Could you check a few things on this model? Use its own coordinates, in mm. Coordinates: 2 decimals unless noted, no trailing zeros. Write each loop counter-clockwise with the first axis right and the second up, starting at its lowest first coordinate (ties: lowest second). Pieces come first, ordered by that corner, then holes.
Autodesk Inventor part; units mm, degrees
ref_plane "YZ Plane" through (0, 0, 0) normal (1, 0, 0) x (0, 1, 0)
ref_plane "XZ Plane" through (0, 0, 0) normal (0, 1, 0) x (-1, 0, 0)
ref_plane "XY Plane" through (0, 0, 0) normal (0, 0, 1) x (1, 0, 0)
sketch "Sketch1" plane through (0, 0, 0) normal (0, 1, 0) x (-1, 0, 0)
  line L0 (2.286, 0) -> (10.414, 0)
  line L1 (12.7, -2.286) -> (12.7, -10.414)
  line L2 (10.414, -12.7) -> (2.286, -12.7)
  line L3 (0, -10.414) -> (0, -2.286)
  line L4 (8.1534, -4.0386) -> (4.5466, -4.0386)
  line L5 (4.0386, -4.5466) -> (4.0386, -8.1534)
  line L6 (4.5466, -8.6614) -> (8.1534, -8.6614)
  line L7 (8.6614, -8.1534) -> (8.6614, -4.5466)
  line L8 (10.414, 0) -> (12.7, -2.286)
  line L9 (12.7, -10.414) -> (10.414, -12.7)
  line L10 (2.286, -12.7) -> (0, -10.414)
  line L11 (2.286, 0) -> (0, -2.286)
  arc A0 (8.6614, -4.5466) -> (8.1534, -4.0386) centre (8.1534, -4.5466) ccw
  arc A1 (8.1534, -8.6614) -> (8.6614, -8.1534) centre (8.1534, -8.1534) ccw
  arc A2 (4.0386, -8.1534) -> (4.5466, -8.6614) centre (4.5466, -8.1534) ccw
  arc A3 (4.5466, -4.0386) -> (4.0386, -4.5466) centre (4.5466, -4.5466) ccw
  line L12 (8.1534, -4.5466) -> (4.5466, -8.1534) construction
  line L13 (12.7, -10.414) -> (0, -2.286) construction
  point P0 (0, 0)
  point P1 (12.7, -12.7)
  point P2 (12.7, 0)
  point P3 (0, -12.7)
  point P4 (4.0386, -8.6614)
  point P5 (8.6614, -8.6614)
  point P6 (6.35, -6.35)
  dimension "d1" = 12.7
  dimension "d2" = 4.6228
  dimension "d3" = 2.286
  dimension "d4" = 2.286
  dimension "d5" = 2.286
  dimension "d6" = 2.286
  dimension "d7" = 2.286
  dimension "d8" = 2.286
  dimension "d9" = 2.286
  dimension "d10" = 2.286
  dimension "d11" = 0.508
extrude "Body" add sketch "Sketch1" along normal blind 1.1906
sketch "Sketch2" plane through (0, 1.1906, 0) normal (0, 1, 0) x (1, 0, 0)
  arc A0 (-8.1534, 8.6614) -> (-8.6614, 8.1534) centre (-8.1534, 8.1534) ccw construction
  arc A1 (-4.5466, 4.0386) -> (-4.0386, 4.5466) centre (-4.5466, 4.5466) ccw construction
  circle A2 centre (-6.35, 6.35) radius 2.1844
  line L0 (-8.1534, 8.1534) -> (-4.5466, 4.5466) construction
  point P0 (0, 0)
  dimension "d14" = 4.3688
surface extrude "Circle" sketch "Sketch2" against normal up to surface (1.1906 mm away) shown yes curves A2
pattern_linear "Rectangular Pattern1" count 3 spacing 12.7 along (0, 0, -1) of "Body", "Circle"
equation "\"d22\" = d19"
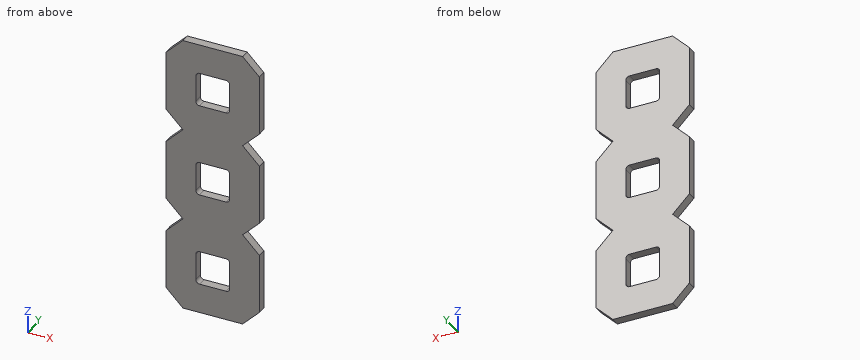
1. I want a section at A-A on x = -5.25. Please give me the cut outline in (y, z).
Verdict:
outline: (0, -38.1) - (1.19, -38.1) - (1.19, -34.06) - (0, -34.06) - close; (0, -29.44) - (1.19, -29.44) - (1.19, -21.36) - (0, -21.36) - close; (0, -16.74) - (1.19, -16.74) - (1.19, -8.66) - (0, -8.66) - close; (0, -4.04) - (1.19, -4.04) - (1.19, 0) - (0, 0) - close
2. I want a section at C-C on x = -10.75. Please give me the cut outline in (y, z).
Verdict:
outline: (0, -37.76) - (1.19, -37.76) - (1.19, -25.74) - (0, -25.74) - close; (0, -25.06) - (1.19, -25.06) - (1.19, -13.04) - (0, -13.04) - close; (0, -12.36) - (1.19, -12.36) - (1.19, -0.34) - (0, -0.34) - close
3. I want a section at B-B on z = -18.5. Please give me the cut outline in (x, y), plus the area to 3 significant figures.
Verdict:
outline: (-12.7, 0) - (-8.66, 0) - (-8.66, 1.19) - (-12.7, 1.19) - close; (-4.04, 0) - (0, 0) - (0, 1.19) - (-4.04, 1.19) - close
area: 9.62 mm2
4. I want a section at D-D on y = 0.45. Give the number of separate pieces and of enclosed holes in the cut face, plus the area to 3 significant figures.
Verdict:
separate pieces: 1
enclosed holes: 3
area: 389 mm2
5. Please list where these lines run through material, in increasing order: line 1 along Z through (x, y) = (-4.75, 1); line 2 along X through (y, z) = (0.5, -8); line 3 along Z through (x, y) = (-0.25, 0.8).
Verdict:
line 1: z = -38.1 to -34.06, -29.44 to -21.36, -16.74 to -8.66, -4.04 to 0
line 2: x = -12.7 to -8.66, -4.04 to 0
line 3: z = -36.06 to -27.44, -23.36 to -14.74, -10.66 to -2.04
